Verification items for the finished model (mm, model axes). Face numbers are marked on the shaded views. Round coordinates to 2 decimals unless told otherwise and drop trailing zeros. Write each loop counter-clockwise with the first axis right and the second up, starting at its lowest first coordinate (ties: lowest second). Pieces come first, ordered by that corner, then holes. Notation, with made-up numbers: M 83,43.5 L 136,43.5 A6 ccw 136,48.5 Z; hole C -27,7 d3. An arc over 180 degrees is marked long. Answer in a Markdown table with one row per item. Add a question column.
1. Sectioned sample at A-A on y = 5. Record the cut outline in (x, z).
2. Sectioned sample at B-B on z = 28.25. Count the separate pieces of the cut face and the enclosed holes in it, plus the area to 3 significant figures.
3. Go/stop test with flat-tipped pins: pin 1 Ø1 at (x, y) = (22.5, 22.5) entering from -Z; pin 2 Ø2 at (x, z) = (101, 23.5) entering from +Y. Record where each tip stops, or that it passes through.
4. Material ranges on probe 1 along Y at (x, z) = (80, 18.5); probe 2 along Y at (x, z) = (5, 23.5); probe 3 along X at (y, z) = (32.5, 22.75), recorded low to high.
5. Draft check along X on the marked faces 1, 2 and 3. Enter one of: pulls with the +X half, pulls with the -X half, needs draft (parallel to the pull), parting line crosses it, or undercut.
```python
from build123d import *

# Parameters (mm, degrees)
SKIZZE2_W                        = 120
SKIZZE2_H                        = 39.364160046
AUFSATZ_LINEAR_AUSTRAGEN1_DEPTH  = 30
SKIZZE24_R                       = 1.55
SCHNITT_LINEAR_AUSTRAGEN4_DEPTH  = 130.805766806
SKIZZE46_R                       = 2.85
SCHNITT_LINEAR_AUSTRAGEN15_DEPTH = 10
SCHNITT_LINEAR_START             = -5
SCHNITT_LINEAR_AUSTRAGEN25_DEPTH = 2.7
LINEARES_MUSTER1_COUNT           = 4
LINEARES_MUSTER1_PITCH           = 20
SPIEGELN2_COPY_1_SKETCH_R        = 2.85
SPIEGELN2_COPY_1_DEPTH           = 10
SPIEGELN2_COPY_2_SKETCH_R        = 2.85
SPIEGELN2_COPY_2_DEPTH           = 10
SPIEGELN2_COPY_3_SKETCH_R        = 2.85
SPIEGELN2_COPY_3_DEPTH           = 10
SPIEGELN2_START                  = -5
SPIEGELN2_COPY_4_DEPTH           = 2.7
SPIEGELN2_COPY_5_DEPTH           = 2.7
SPIEGELN2_COPY_6_DEPTH           = 2.7
SKIZZE51_R                       = 1.55
SCHNITT_LINEAR_AUSTRAGEN26_DEPTH = 130.805766806
SKIZZE75_R                       = 0.75
SCHNITT_LINEAR_AUSTRAGEN28_DEPTH = 10
SKIZZE76_R                       = 2
SCHNITT_LINEAR_AUSTRAGEN29_DEPTH = 6
SKIZZE80_R                       = 0.5
SCHNITT_LINEAR_AUSTRAGEN34_DEPTH = 21
SCHNITT_LINEAR_START_2           = -7.5
SKIZZE81_R                       = 0.5
SCHNITT_LINEAR_AUSTRAGEN36_DEPTH = 5
ABSPALTEN3_OUTLINE_W             = 120
ABSPALTEN3_OUTLINE_H             = 39.364160046
ABSPALTEN3_OUTLINE_R             = 1.55
ABSPALTEN3_DEPTH                 = 15


# Read off the part's stored shape, not the designer's step: Abspalten3
with BuildPart() as part:
    # Skizze2 → Aufsatz-Linear austragen1 (new body)
    with BuildSketch(Plane.XY):
        with Locations((60, 19.682080023)):
            Rectangle(SKIZZE2_W, SKIZZE2_H)
    extrude(amount=AUFSATZ_LINEAR_AUSTRAGEN1_DEPTH)

    # Skizze24 → Schnitt-Linear austragen4 (cut, through all)
    with BuildSketch(Plane.XY.offset(30)):
        with Locations((40, 31.364160046)):
            Circle(SKIZZE24_R)
        with Locations((60, 31.364160046)):
            Circle(SKIZZE24_R)
        with Locations((80, 31.364160046)):
            Circle(SKIZZE24_R)
        with Locations((100, 31.364160046)):
            Circle(SKIZZE24_R)
    schnitt_linear_austragen4 = extrude(amount=-SCHNITT_LINEAR_AUSTRAGEN4_DEPTH, mode=Mode.SUBTRACT)

    # Skizze46 → Schnitt-Linear austragen15 (cut)
    with BuildSketch(Plane(origin=(0, 0, 0), x_dir=(-1, 0, 0), z_dir=(0, 0, -1))):
        with Locations((-100, 31.364160046)):
            Circle(SKIZZE46_R)
    schnitt_linear_austragen15 = extrude(amount=-SCHNITT_LINEAR_AUSTRAGEN15_DEPTH, mode=Mode.SUBTRACT)

    # Skizze50 → Schnitt-Linear austragen25 (cut)
    with BuildSketch(Plane.XY.offset(30).offset(SCHNITT_LINEAR_START)):
        Polygon((97.15, 33.009608314), (97.15, 39.364160046), (102.85, 39.364160046), (102.85, 33.009608314), (102.85, 29.718711779), (100, 28.073263512), (97.15, 29.718711779), align=None)
    schnitt_linear_austragen25 = extrude(amount=-SCHNITT_LINEAR_AUSTRAGEN25_DEPTH, mode=Mode.SUBTRACT)

    # Lineares Muster1: Schnitt-Linear austragen15, Schnitt-Linear austragen25 ×4
    with Locations(*[(-i * LINEARES_MUSTER1_PITCH, 0, 0) for i in range(1, LINEARES_MUSTER1_COUNT)]):
        add(schnitt_linear_austragen15, mode=Mode.SUBTRACT)
        add(schnitt_linear_austragen25, mode=Mode.SUBTRACT)

    # Spiegeln2: Schnitt-Linear austragen15, Schnitt-Linear austragen25 across plane
    add(schnitt_linear_austragen15.mirror(Plane.ZX.offset(19.764160046)), mode=Mode.SUBTRACT)
    add(schnitt_linear_austragen25.mirror(Plane.ZX.offset(19.764160046)), mode=Mode.SUBTRACT)

    # Spiegeln2 copy 1 sketch → Spiegeln2 copy 1 (cut)
    with BuildSketch(Plane(origin=(-20, 39.528320093, 0), x_dir=(-1, 0, 0), z_dir=(0, 0, -1))):
        with Locations((-100, -31.364160046)):
            Circle(SPIEGELN2_COPY_1_SKETCH_R)
    extrude(amount=-SPIEGELN2_COPY_1_DEPTH, mode=Mode.SUBTRACT)

    # Spiegeln2 copy 2 sketch → Spiegeln2 copy 2 (cut)
    with BuildSketch(Plane(origin=(-40, 39.528320093, 0), x_dir=(-1, 0, 0), z_dir=(0, 0, -1))):
        with Locations((-100, -31.364160046)):
            Circle(SPIEGELN2_COPY_2_SKETCH_R)
    extrude(amount=-SPIEGELN2_COPY_2_DEPTH, mode=Mode.SUBTRACT)

    # Spiegeln2 copy 3 sketch → Spiegeln2 copy 3 (cut)
    with BuildSketch(Plane(origin=(-60, 39.528320093, 0), x_dir=(-1, 0, 0), z_dir=(0, 0, -1))):
        with Locations((-100, -31.364160046)):
            Circle(SPIEGELN2_COPY_3_SKETCH_R)
    extrude(amount=-SPIEGELN2_COPY_3_DEPTH, mode=Mode.SUBTRACT)

    # Spiegeln2 copy 4 sketch → Spiegeln2 copy 4 (cut)
    with BuildSketch(Plane(origin=(-20, 39.528320093, 30), x_dir=(1, 0, 0), z_dir=(0, 0, 1)).offset(SPIEGELN2_START)):
        Polygon((97.15, -33.009608314), (97.15, -39.364160046), (102.85, -39.364160046), (102.85, -33.009608314), (102.85, -29.718711779), (100, -28.073263512), (97.15, -29.718711779), align=None)
    extrude(amount=-SPIEGELN2_COPY_4_DEPTH, mode=Mode.SUBTRACT)

    # Spiegeln2 copy 5 sketch → Spiegeln2 copy 5 (cut)
    with BuildSketch(Plane(origin=(-40, 39.528320093, 30), x_dir=(1, 0, 0), z_dir=(0, 0, 1)).offset(SPIEGELN2_START)):
        Polygon((97.15, -33.009608314), (97.15, -39.364160046), (102.85, -39.364160046), (102.85, -33.009608314), (102.85, -29.718711779), (100, -28.073263512), (97.15, -29.718711779), align=None)
    extrude(amount=-SPIEGELN2_COPY_5_DEPTH, mode=Mode.SUBTRACT)

    # Spiegeln2 copy 6 sketch → Spiegeln2 copy 6 (cut)
    with BuildSketch(Plane(origin=(-60, 39.528320093, 30), x_dir=(1, 0, 0), z_dir=(0, 0, 1)).offset(SPIEGELN2_START)):
        Polygon((97.15, -33.009608314), (97.15, -39.364160046), (102.85, -39.364160046), (102.85, -33.009608314), (102.85, -29.718711779), (100, -28.073263512), (97.15, -29.718711779), align=None)
    extrude(amount=-SPIEGELN2_COPY_6_DEPTH, mode=Mode.SUBTRACT)

    # Spiegeln3: Schnitt-Linear austragen4 across plane
    add(schnitt_linear_austragen4.mirror(Plane.ZX.offset(19.764160046)), mode=Mode.SUBTRACT)

    # Skizze51 → Schnitt-Linear austragen26 (cut, through all)
    with BuildSketch(Plane.XY.offset(30)):
        with Locations((5, 34.364160046)):
            Circle(SKIZZE51_R)
        with Locations((115, 5)):
            Circle(SKIZZE51_R)
    extrude(amount=-SCHNITT_LINEAR_AUSTRAGEN26_DEPTH, mode=Mode.SUBTRACT)

    # Skizze73 → Schnitt-Rotation5 (revolve, cut)
    with BuildSketch(Plane.XY.offset(15)):
        Polygon((15, 19.764160046), (15, 23.264160046), (20, 23.264160046), (20, 24.264160046), (100, 22.682080023), (100, 21.682080023), (105, 21.682080023), (105, 19.682080023), align=None)
    revolve(axis=Axis((105, 19.682080023, 15), (-0.9999995841280241, 0.0009119998787298228, 0)), mode=Mode.SUBTRACT)

    # Skizze75 → Schnitt-Linear austragen28 (cut)
    with BuildSketch(Plane.XY.offset(30)):
        with Locations((21.598259807, 19.682080023)):
            Circle(SKIZZE75_R)
    extrude(amount=-SCHNITT_LINEAR_AUSTRAGEN28_DEPTH, mode=Mode.SUBTRACT)

    # Skizze76 → Schnitt-Linear austragen29 (cut)
    with BuildSketch(Plane.XY.offset(30)):
        with Locations((21.598259807, 19.682080023)):
            Circle(SKIZZE76_R)
    extrude(amount=-SCHNITT_LINEAR_AUSTRAGEN29_DEPTH, mode=Mode.SUBTRACT)

    # Skizze80 → Schnitt-Linear austragen34 (cut)
    with BuildSketch(Plane(origin=(120, 0, 0), x_dir=(0, 0, -1), z_dir=(1, 0, 0))):
        with Locations((-22.000416524, 19.763714623)):
            Circle(SKIZZE80_R)
    schnitt_linear_austragen34 = extrude(amount=-SCHNITT_LINEAR_AUSTRAGEN34_DEPTH, mode=Mode.SUBTRACT)

    # Skizze81 → Schnitt-Linear austragen36 (cut)
    with BuildSketch(Plane.XY.offset(30).offset(SCHNITT_LINEAR_START_2)):
        with Locations(Location((99, 19.682080023, 0), (0, 0, 7.034090001))):
            Circle(SKIZZE81_R)
    schnitt_linear_austragen36 = extrude(amount=-SCHNITT_LINEAR_AUSTRAGEN36_DEPTH, mode=Mode.SUBTRACT)

    # Spiegeln4: Schnitt-Linear austragen34, Schnitt-Linear austragen36 across plane
    add(schnitt_linear_austragen34.mirror(Plane.XY.offset(15)), mode=Mode.SUBTRACT)
    add(schnitt_linear_austragen36.mirror(Plane.XY.offset(15)), mode=Mode.SUBTRACT)

    # Abspalten3 outline → Abspalten3 (cut)
    with BuildSketch(Plane.XY):
        with Locations((60, 19.682080023)):
            Rectangle(ABSPALTEN3_OUTLINE_W, ABSPALTEN3_OUTLINE_H)
        with Locations((115, 5)):
            Circle(ABSPALTEN3_OUTLINE_R, mode=Mode.SUBTRACT)
        with Locations((5, 34.364160046)):
            Circle(ABSPALTEN3_OUTLINE_R, mode=Mode.SUBTRACT)
        with Locations((40, 8.164160046)):
            Circle(ABSPALTEN3_OUTLINE_R, mode=Mode.SUBTRACT)
        with Locations((60, 8.164160046)):
            Circle(ABSPALTEN3_OUTLINE_R, mode=Mode.SUBTRACT)
        with Locations((80, 8.164160046)):
            Circle(ABSPALTEN3_OUTLINE_R, mode=Mode.SUBTRACT)
        with Locations((100, 8.164160046)):
            Circle(ABSPALTEN3_OUTLINE_R, mode=Mode.SUBTRACT)
        with Locations((40, 31.364160046)):
            Circle(ABSPALTEN3_OUTLINE_R, mode=Mode.SUBTRACT)
        with Locations((100, 31.364160046)):
            Circle(ABSPALTEN3_OUTLINE_R, mode=Mode.SUBTRACT)
        with Locations((60, 31.364160046)):
            Circle(ABSPALTEN3_OUTLINE_R, mode=Mode.SUBTRACT)
        with Locations((80, 31.364160046)):
            Circle(ABSPALTEN3_OUTLINE_R, mode=Mode.SUBTRACT)
    extrude(amount=ABSPALTEN3_DEPTH, mode=Mode.SUBTRACT)


solid = part.part
```
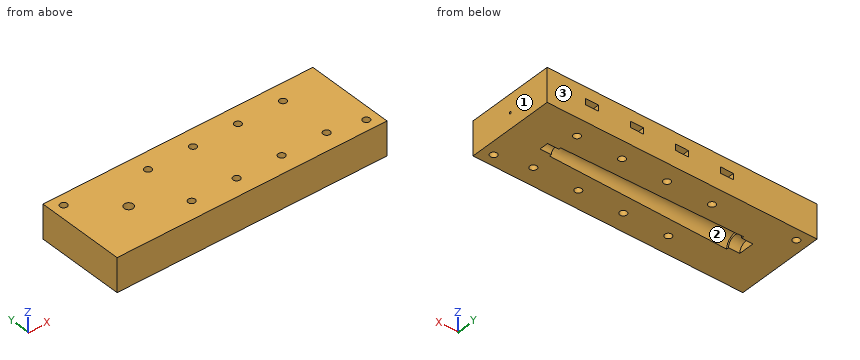
Geometry check:
| question | item | result |
|---|---|---|
| 1 | outline | M 0,15 L 113.45,15 L 113.45,30 L 0,30 Z; M 116.55,15 L 120,15 L 120,30 L 116.55,30 Z; hole M 37.15,22.3 L 42.85,22.3 L 42.85,25 L 37.15,25 Z; hole M 57.15,22.3 L 62.85,22.3 L 62.85,25 L 57.15,25 Z; hole M 77.15,22.3 L 82.85,22.3 L 82.85,25 L 77.15,25 Z; hole M 97.15,22.3 L 102.85,22.3 L 102.85,25 L 97.15,25 Z |
| 2 | separate pieces | 1 |
| 2 | enclosed holes | 11 |
| 2 | area | 4,640 mm2 |
| 3 | pin 1 | stops at z = 18.06 |
| 3 | pin 2 | stops at y = 29.23 |
| 4 | probe 1 | y = 0 to 6.61, 9.71 to 29.81, 32.91 to 39.36 |
| 4 | probe 2 | y = 0 to 32.81, 35.91 to 39.36 |
| 4 | probe 3 | x = 0 to 37.15, 42.85 to 57.15, 62.85 to 77.15, 82.85 to 97.15, 102.85 to 120 |
| 5 | face 1 | pulls with the +X half |
| 5 | face 2 | undercut |
| 5 | face 3 | needs draft |
